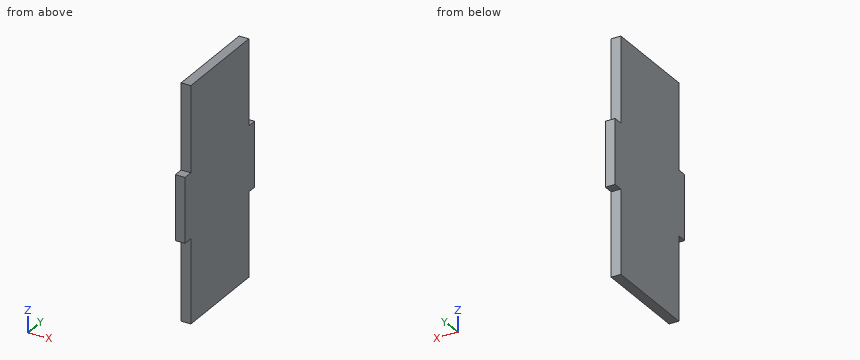
from build123d import *

# Parameters (mm, degrees)
SKETCH1_W           = 3
SKETCH1_H           = 20
BOSS_EXTRUDE1_DEPTH = 3
SKETCH2_W           = 3
SKETCH2_H           = 72.31
BOSS_EXTRUDE2_DEPTH = 30
SKETCH3_W           = 3
SKETCH3_H           = 20
BOSS_EXTRUDE3_DEPTH = 3


with BuildPart() as part:
    # Sketch1 → Boss-Extrude1 (new body)
    with BuildSketch(Plane(origin=(0, 0, 0), x_dir=(1, 0, 0), z_dir=(0, 1, 0))):
        with Locations((-4.820734675, -44.391585228)):
            Rectangle(SKETCH1_W, SKETCH1_H)
    extrude(amount=BOSS_EXTRUDE1_DEPTH)

    # Sketch2 → Boss-Extrude2 (add)
    with BuildSketch(Plane(origin=(0, 3, 0), x_dir=(1, 0, 0), z_dir=(0, 1, 0))):
        with Locations((-4.820734675, -44.66687809)):
            Rectangle(SKETCH2_W, SKETCH2_H)
    extrude(amount=BOSS_EXTRUDE2_DEPTH)

    # Sketch3 → Boss-Extrude3 (add)
    with BuildSketch(Plane(origin=(0, 33, 0), x_dir=(1, 0, 0), z_dir=(0, 1, 0))):
        with Locations((-4.820734675, -44.391585228)):
            Rectangle(SKETCH3_W, SKETCH3_H)
    extrude(amount=BOSS_EXTRUDE3_DEPTH)


solid = part.part
Here's how the part is built. I have some questions about the finished solid (model axes, mm). Round coordinates to 2 decimals unless told otherwise and drop trailing zeros. Loops run counter-clockwise (first coordinate to the right, second up) from the corner with the lowest first, then second, coordinate; pieces in that order, holes last.
1. If I drill on line 1 along Y through (x, z) = (-5.15, 62.5), over which ranges is the centre line in solid material (lowest first)?
Answer list:
line 1: y = 3 to 33
2. For P1, Ø1.5, axis at x = -5, z = 26, coming from the +Y side; P2, Ø0.9, axis at x = -5, y = 34.5, coming from the +Z side, each with a flat end and sliding along its axis, tell me the tip position at first contact or that it passes through.
Answer list:
P1: stops at y = 33
P2: stops at z = 54.39
3. If we section it at B-B on z = 65: Write out the boundary of the cut face in (x, y), plus the area to 3 significant figures.
Answer list:
outline: (-6.32, 3) - (-3.32, 3) - (-3.32, 33) - (-6.32, 33) - close
area: 90.0 mm2
4. If we section it at A-A on x = -5.35: Write out the boundary of the cut face in (y, z).
Answer list:
outline: (0, 34.39) - (3, 34.39) - (3, 8.51) - (33, 8.51) - (33, 34.39) - (36, 34.39) - (36, 54.39) - (33, 54.39) - (33, 80.82) - (3, 80.82) - (3, 54.39) - (0, 54.39) - close
